Geometry: final body of the model. Coordinates: model frame, mm. Round coordinates to 2 decimals unless told otherwise and drop trailing zeros. Loops run counter-clockwise (first coordinate to the right, second up) from the corner with the lowest first, then second, coordinate; pieces in that order, holes last. Notation, with made-up numbers: (-39, 4) - (-13, 4) arc R38 ccw to (-13, 42) - close; hole circle Ø9 at (31.25, 49.5). An arc over 180 degrees is marked (long way). Answer as a JSON object with one key per item and string values. Group by question number.
Item 1: Section A-A (z = -5). Return the cut outline in (x, y).
Item 2: Section B-B (y = 0.9). Return the cut outline in (x, z), plus the area to 3 significant figures.
Item 3: Line query: line 1 (Z direction, x = 160.5, y = 0.9); line 2 (X direction, y = 1.6, z = -5); line 3 (Z direction, x = 120, y = 1.3). Output: solid intervals per line, ascending.
Item 4: Section C-C (x = 143.5). Return the cut outline in (y, z).
Item 5: Draft query along Z for faces 1 (the face through (164.083, 1, 11)), 2 (the face through (121.13, 0.89, -5.44)). Return one class per face: released by +Z, released by -Z, zero draft, split by the parting line, or undercut.
Item 6: First-contact query: pin 1 (0.9 mm diameter, centred on x = 95, y = 1, fed in from +Z); pin 2 (0.9 mm diameter, centred on x = 149.5, y = 1, fed in from -Z). Flat tips, straight axial feed; report the tip coordinate or a pass-through.
Item 7: Section D-D (z = 27). Return the cut outline in (x, y).
```python
from build123d import *

# Parameters (mm, degrees)
SKETCH1_R           = 2
BOSS_EXTRUDE1_DEPTH = 1.8


with BuildPart() as part:
    # Sketch1 → Boss-Extrude1 (new body)
    with BuildSketch(Plane(origin=(0, 0, 0), x_dir=(1, 0, 0), z_dir=(0, 1, 0))):
        with BuildLine():
            Line((118.18380357, 2.009694076), (82.082783055, 2.009694076))
            Line((82.082783055, 2.009694076), (82.082783055, -23.990305924))
            Line((82.082783055, -23.990305924), (118.18380357, -23.990305924))
            ThreePointArc((118.18380357, -23.990305924), (123.082783055, -29.990305924), (127.981762541, -23.990305924))
            Line((127.981762541, -23.990305924), (164.082783055, -23.990305924))
            Line((164.082783055, -23.990305924), (164.082783055, 2.009694076))
            Line((164.082783055, 2.009694076), (127.981762541, 2.009694076))
            ThreePointArc((127.981762541, 2.009694076), (123.082783055, 8.009694076), (118.18380357, 2.009694076))
        make_face()
        with Locations(Location((123.082783055, 5.009694076, 0), (0, 0, 270))):
            Circle(SKETCH1_R, mode=Mode.SUBTRACT)
        with Locations(Location((123.082783055, -26.990305924, 0), (0, 0, 270))):
            Circle(SKETCH1_R, mode=Mode.SUBTRACT)
    extrude(amount=BOSS_EXTRUDE1_DEPTH)


solid = part.part
```
Values:
{
 "1": {"outline": "(118.5, 0) - (121.08, 0) - (121.08, 1.8) - (118.5, 1.8) - close; (125.08, 0) - (127.67, 0) - (127.67, 1.8) - (125.08, 1.8) - close"},
 "2": {"outline": "(82.08, -2.01) - (118.18, -2.01) arc R5 ccw (long way) to (127.98, -2.01) - (164.08, -2.01) - (164.08, 23.99) - (127.98, 23.99) arc R5 ccw (long way) to (118.18, 23.99) - (82.08, 23.99) - close; hole circle Ø4 at (123.08, -5.01); hole circle Ø4 at (123.08, 26.99)", "area": "2,210 mm^2"},
 "3": {"line 1": "z = -2.01 to 23.99", "line 2": "x = 118.5 to 121.08, 125.08 to 127.67", "line 3": "z = -6.95 to 28.93"},
 "4": {"outline": "(0, -2.01) - (1.8, -2.01) - (1.8, 23.99) - (0, 23.99) - close"},
 "5": {"face 1": "zero draft", "face 2": "undercut"},
 "6": {"pin 1": "stops at z = 23.99", "pin 2": "stops at z = -2.01"},
 "7": {"outline": "(118.5, 0) - (121.08, 0) - (121.08, 1.8) - (118.5, 1.8) - close; (125.08, 0) - (127.66, 0) - (127.66, 1.8) - (125.08, 1.8) - close"}
}
